Source: CAD feature listing. Evaluate the final solid. Frame: model axes, mm. A direction names the side the tool comes from. Give positions to 0.01 mm unless a question says otherwise; leave off trailing zeros. Loops run counter-clockwise (first coordinate to the right, second up) from the corner with the lowest first, then second, coordinate; pieces in that order, holes last.
from build123d import *

# Parameters (mm, degrees)
SKETCH001_R   = 6.985
SKETCH001_R_2 = 11.176
SKETCH001_R_3 = 6.35
SKETCH001_R_4 = 6.477
SKETCH001_R_5 = 2
SKETCH001_R_6 = 2.5
SKETCH001_R_7 = 13.85
PAD_DEPTH     = 12.999999
SKETCH_R      = 2.54
POCKET_DEPTH  = 20.32


with BuildPart() as part:
    # Sketch001 → Pad (new body)
    with BuildSketch(Plane.XY):
        with BuildLine():
            Line((0, 0), (304.8, 0))
            Line((304.8, 127), (304.8, 0))
            ThreePointArc((304.8, 127), (301.080256, 135.980256), (292.1, 139.7))
            Line((12.7, 139.7), (292.1, 139.7))
            ThreePointArc((12.7, 139.7), (3.719744, 135.980256), (0, 127))
            Line((0, 0), (0, 127))
        make_face()
        with Locations((285.75, 88.9)):
            Circle(SKETCH001_R, mode=Mode.SUBTRACT)
        with Locations((133.35, 76.2)):
            Circle(SKETCH001_R_2, mode=Mode.SUBTRACT)
        with Locations((25.4, 19.05)):
            Circle(SKETCH001_R_3, mode=Mode.SUBTRACT)
        with Locations((101.6, 19.05)):
            Circle(SKETCH001_R_3, mode=Mode.SUBTRACT)
        with Locations((254, 19.05)):
            Circle(SKETCH001_R_3, mode=Mode.SUBTRACT)
        with Locations((133.35, 19.05)):
            Circle(SKETCH001_R_4, mode=Mode.SUBTRACT)
        with Locations((30.1625, 88.9)):
            Circle(SKETCH001_R_2, mode=Mode.SUBTRACT)
        with Locations((14.6625, 73.4)):
            Circle(SKETCH001_R_5, mode=Mode.SUBTRACT)
        with Locations((45.6625, 104.4)):
            Circle(SKETCH001_R_5, mode=Mode.SUBTRACT)
        with Locations((45.6625, 73.4)):
            Circle(SKETCH001_R_5, mode=Mode.SUBTRACT)
        with Locations((14.6625, 104.4)):
            Circle(SKETCH001_R_5, mode=Mode.SUBTRACT)
        with Locations((117.85, 91.7)):
            Circle(SKETCH001_R_5, mode=Mode.SUBTRACT)
        with Locations((148.85, 91.7)):
            Circle(SKETCH001_R_5, mode=Mode.SUBTRACT)
        with Locations((117.85, 60.7)):
            Circle(SKETCH001_R_5, mode=Mode.SUBTRACT)
        with Locations((148.85, 60.7)):
            Circle(SKETCH001_R_5, mode=Mode.SUBTRACT)
        with Locations((177.8, 19.05)):
            Circle(SKETCH001_R_6, mode=Mode.SUBTRACT)
        with Locations((177.8, 50.8)):
            Circle(SKETCH001_R_6, mode=Mode.SUBTRACT)
        with Locations((69.85, 114.3)):
            Circle(SKETCH001_R_7, mode=Mode.SUBTRACT)
        with Locations((85.588112, 75.00004)):
            Circle(SKETCH001_R_7, mode=Mode.SUBTRACT)
        with Locations((114.000062, 114.3)):
            Circle(SKETCH001_R_7, mode=Mode.SUBTRACT)
        with Locations((153.610092, 114.3)):
            Circle(SKETCH001_R_7, mode=Mode.SUBTRACT)
    extrude(amount=PAD_DEPTH)

    # Sketch → Pocket (cut)
    with BuildSketch(Plane.XZ):
        with Locations((25.4, 6.5)):
            Circle(SKETCH_R)
        with Locations((101.6, 6.5)):
            Circle(SKETCH_R)
        with Locations((254, 6.5)):
            Circle(SKETCH_R)
    extrude(amount=-POCKET_DEPTH, mode=Mode.SUBTRACT)


solid = part.part
1) Contact query for a flat-ended pin moving along its axis: P1, Ø5, axis at x = 45.66, y = 104.4, coming from the -Z side. Output: stop coordinate, or through.
Checks:
P1: stops at z = 0
2) Ray query, probe 1 along X at (y, z) = (9.5, 6.5); probe 2 along Y at (x, z) = (46, 12.25); probe 3 along Y at (x, z) = (177.8, 3.5). Return the intervals inside material, ascending.
Checks:
probe 1: x = 0 to 22.86, 27.94 to 99.06, 104.14 to 251.46, 256.54 to 304.8
probe 2: y = 0 to 71.43, 75.37 to 102.43, 106.37 to 139.7
probe 3: y = 0 to 16.55, 21.55 to 48.3, 53.3 to 139.7
3) Pull-direction query (X, two-part tool) for faces 1 (the cylindrical face through (111, 100.78, 6.41)), 2 (the flat face through (0, 63, 6)), 3 (the cylindrical face through (292.41, 91, 6.41)), 4 (the flat face through (150, 139.7, 6)); classes: released by +X, released by -X, zero draft, split by the parting line, or undercut.
Checks:
face 1: undercut
face 2: released by -X
face 3: undercut
face 4: zero draft
4) Cut plane A-A (x = 133.35). Return loops of the section in (y, z), and give its area (3 significant figures).
Checks:
outline: (0, 0) - (12.57, 0) - (12.57, 13) - (0, 13) - close; (25.53, 0) - (65.02, 0) - (65.02, 13) - (25.53, 13) - close; (87.38, 0) - (139.7, 0) - (139.7, 13) - (87.38, 13) - close
area: 1,360 mm2
5) Cut plane B-B (y = 111). Return loops of the section in (x, z), and give its area (3 significant figures).
Checks:
outline: (0, 0) - (56.4, 0) - (56.4, 13) - (0, 13) - close; (83.3, 0) - (100.55, 0) - (100.55, 13) - (83.3, 13) - close; (127.45, 0) - (140.16, 0) - (140.16, 13) - (127.45, 13) - close; (167.06, 0) - (304.8, 0) - (304.8, 13) - (167.06, 13) - close
area: 2,910 mm2
6) Reachability of faces 5 (the flat face through (150, 71, 0)), 6 (the cylindrical face through (256.346, 6.522, 5.527)) from +Z, -Z, +X, -X, +Y, -Y: full face, straight path, thin tool, end or side. Return the list, or none.
Checks:
face 5: -Z, +X, -X, +Y, -Y
face 6: -Y
